```python
from build123d import *

# Parameters (mm, degrees)
F0_R     = 41.275
F0_R_2   = 31.75
F1_DEPTH = 15.875
F2_R     = 41.275
F3_DEPTH = 34.925
F4_R     = 12.7
F5_DEPTH = 50.8


with BuildPart() as f1:
    # F0 (on Top) → F1 (new body)
    with BuildSketch(Plane.XY):
        Circle(F0_R)
        Circle(F0_R_2, mode=Mode.SUBTRACT)
    extrude(amount=F1_DEPTH)

    # F2 (on face) → F3 (join)
    with BuildSketch(Plane.XY):
        Circle(F2_R)
    extrude(amount=-F3_DEPTH)

    # F4 (on face) → F5 (cut)
    with BuildSketch(Plane(origin=(0, 0, -34.925), x_dir=(1, 0, 0), z_dir=(0, 0, -1))):
        Circle(F4_R)
    extrude(amount=-F5_DEPTH, mode=Mode.SUBTRACT)


solid = f1.part
```
CAD build for the part. Positions are in the model's coordinates, mm. A direction names the side the tool comes from. Coordinates: 2 decimals unless noted, no trailing zeros. Write each loop counter-clockwise with the first axis right and the second up, starting at its lowest first coordinate (ties: lowest second). Pieces come first, ordered by that corner, then holes.
(1) Cut at A-A, the plane x = 0. List the corners of the cut face in (y, z) (3 decimals).
(2) Flat gauge pins, fed straight in: pin 1 (1.5 mm diameter, centred on x = -14, z = -13, fed in from -Y); pin 2 (1 mm diameter, centred on x = 23, z = 4.5, fed in from -Y); pin 3 (10 mm diameter, centred on y = 29, z = -29, fed in from +X); pin 4 (10 mm diameter, centred on x = 3.5, y = -2, fed in from +Z). Where does each tip first touch, or does it go through?
(3) 3-axis set-ups, long thin cutter, end or side, ignore diameter. For faces 1 (the face through (-2.75, 12.4, -17.71)), 2 (the face through (-6.883, -30.995, 7.826)): which of +Z, -Z, +X, -X, +Y, -Y reach the whole face in a straight line?
(4) Cut at C-C, the plane z = -9. List the corners of the cut face in (x, y) (3 decimals), and give its area (3 significant figures).
(5) Cut at D-D, the plane x = 26. List the corners of the cut face in (y, z) (3 decimals), and give its area (3 significant figures).
(6) Drill centre lines: probe 1 along Y at (x, z) = (0, -26) (3 decimals); probe 2 along Y at (x, z) = (0, 4) (3 decimals); probe 3 along Z at (x, y) = (-13, 13.5) (3 decimals). Where is each one in solid material? Low to high.
(7) Two-plate mould, pull along Y, no slides. Class faces 3 (the face through (-8.948, -40.293, -9.169)), 4 (the face through (14, 0, 0)), 5 (the face through (21.2, -24.3, 15.875)): +Y half, -Y half, draft (parallel to the pull), parting line (faces both ways), or undercut.
Geometry says:
1. outline: (-41.275, -34.925) - (-12.7, -34.925) - (-12.7, 0) - (-31.75, 0) - (-31.75, 15.875) - (-41.275, 15.875) - close; (12.7, -34.925) - (41.275, -34.925) - (41.275, 15.875) - (31.75, 15.875) - (31.75, 0) - (12.7, 0) - close
2. pin 1: stops at y = -39.09
2. pin 2: stops at y = -34.6
2. pin 3: stops at x = 33.58
2. pin 4: passes through
3. face 1: +Z, -Z
3. face 2: +Z
4. outline: circle Ø82.55 at (0, 0); hole circle Ø25.4 at (0, 0)
4. area: 4,850 mm2
5. outline: (-32.057, -34.925) - (32.057, -34.925) - (32.057, 15.875) - (18.223, 15.875) - (18.223, 0) - (-18.223, 0) - (-18.223, 15.875) - (-32.057, 15.875) - close
5. area: 2,680 mm2
6. probe 1: y = -41.275 to -12.7, 12.7 to 41.275
6. probe 2: y = -41.275 to -31.75, 31.75 to 41.275
6. probe 3: z = -34.925 to 0
7. face 3: parting line
7. face 4: undercut
7. face 5: draft
